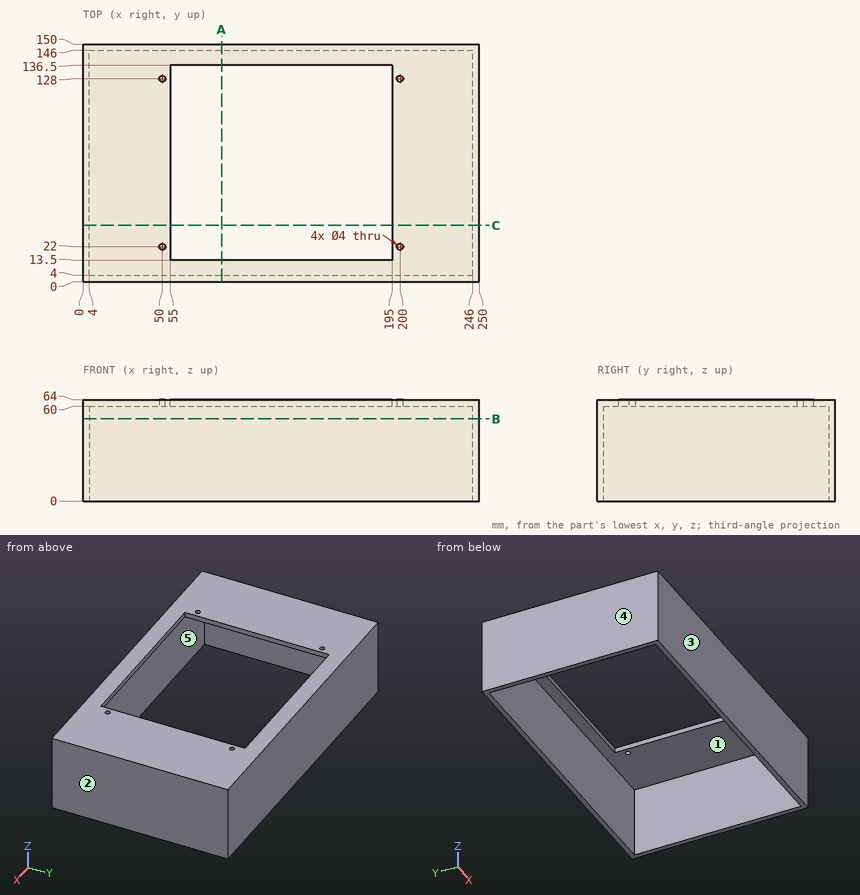
Job drawing, mm, ordinate dimensions from the low corner. One solid piece. A direction names the side the tool comes from. Coordinates: 2 decimals unless noted, no trailing zeros. Order: outer loops, then holes, each group sorted by start corner. A loop starts at its lowest first (then second) coordinate and runs counter-clockwise, first axis right, second up. Notation, with made-up numbers: (29.25, 2) - (73.25, 2) arc R30 ccw to (73.25, 32) - close; hole circle Ø5 at (46.25, -19). An arc over 180 degrees is marked (long way). Use CSV: the item, a comma, the result in double quotes.
Item 1: Probe probe 1 along X at (y, z) = (22, 60.8); probe 2 along Y at (x, z) = (200, 61); probe 3 along X at (y, z) = (112, 18.5). List the from-to ranges inside material, lowest first.
Solved:
probe 1,"x = 0 to 48, 52 to 55, 195 to 198, 202 to 250"
probe 2,"y = 0 to 20, 24 to 126, 130 to 150"
probe 3,"x = 0 to 4, 246 to 250"
Item 2: Mould opens along Y. For the marked faces 1, 2 and 3 say: +Y half, -Y half, draft (parallel to the pull), parting line (faces both ways), or undercut.
Solved:
face 1,"undercut"
face 2,"draft"
face 3,"-Y half"
Item 3: 3-axis set-ups, long thin cutter, end or side, ignore diameter. For the marked faces 4 and 5: which of +Z, -Z, +X, -X, +Y, -Y reach the whole face in a straight line?
Solved:
face 4,"+Z, -Z, -X, +Y, -Y"
face 5,"-Z"
Item 4: Drop flat-ended pins along their axis: P1, Ø4.5, axis at x = 200, y = 128, coming from the -Z side; P2, Ø2.5, axis at x = 50, y = 22, coming from the -Z side. Give the stop position or say it passes through.
Solved:
P1,"stops at z = 60"
P2,"passes through"
Item 5: Saw through at B-B on z = 52. Give the cut face in (x, y).
Solved:
outline,"(0, 0) - (250, 0) - (250, 150) - (0, 150) - close; hole (4, 4) - (246, 4) - (246, 146) - (4, 146) - close"
Item 6: Saw through at C-C on y = 35.5. Give the cut face in (x, z).
Solved:
outline,"(0, 0) - (4, 0) - (4, 60) - (55, 60) - (55, 64) - (0, 64) - close; (195, 60) - (246, 60) - (246, 0) - (250, 0) - (250, 64) - (195, 64) - close"
Item 7: Saw through at A-A on x = 87.5. Give the cut face in (y, z), and give its area (3 significant figures).
Solved:
outline,"(0, 0) - (4, 0) - (4, 60) - (13.5, 60) - (13.5, 64) - (0, 64) - close; (136.5, 60) - (146, 60) - (146, 0) - (150, 0) - (150, 64) - (136.5, 64) - close"
area,"588 mm²"
